Study the drawing (mm; zero at the part's minimum x, y, z) and answer. Give positions to 0.01 mm unless a question says otherwise; leave off trailing zeros. Order: outer loops, then holes, each group sorted by start corner. A loop starts at its lowest first (then second) coordinate and runs counter-clockwise, first axis right, second up. Notation, with made-up numbers: (0, 47) -> (19, 47) arc R25 cw to (19, 80) -> close; hole circle Ø2 at (-6.5, -3). An arc over 180 degrees is marked (long way). Answer as CSV lines item,"result". Start each with the question number.
1. A cutting plane is placed at A-A (y = 3.75). Give the vertices of the cut face in (x, z) (1 decimal).
2. Find the intervals of material crossed by L1, parallel to X at y = 5, z = 1.25; L2, parallel to Y at x = 2, z = 7.5 (1 decimal); L3, parallel to Y at x = 1, z = 2 (1 decimal), in increasing order.
3. A cutting plane is placed at D-D (y = 5.25). Give the vertices of the cut face in (x, z).
4. A cutting plane is placed at B-B (x = 9). Give the vertices of the cut face in (y, z) (1 decimal).
5. A cutting plane is placed at C-C (z = 8.25). Give the vertices of the cut face in (x, y) (1 decimal).
6. For a pull along X with two mould halves and no side action, classify the marked faces 1, 2 and 3 as released by +X, released by -X, zero draft, split by the parting line, or undercut.
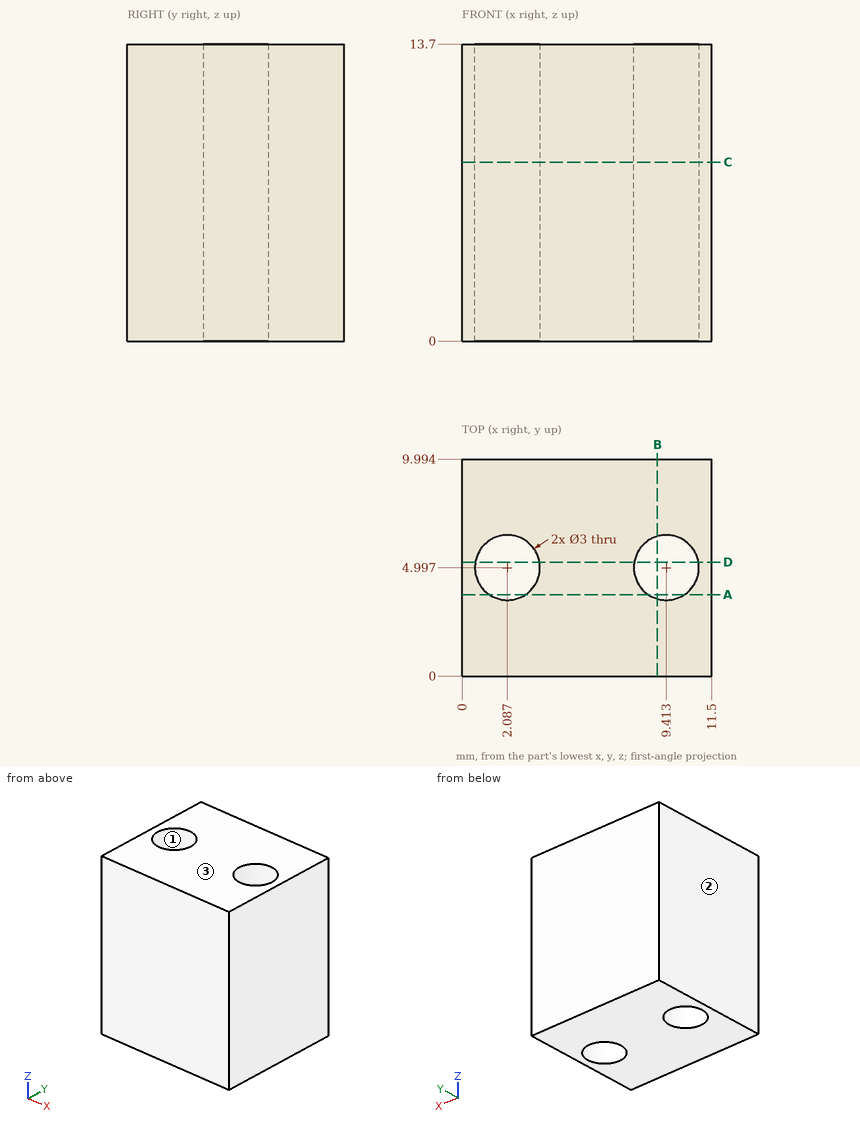
Answer sheet:
1,outline,"(0, 0) -> (1.3, 0) -> (1.3, 13.7) -> (0, 13.7) -> close; (2.9, 0) -> (8.6, 0) -> (8.6, 13.7) -> (2.9, 13.7) -> close; (10.2, 0) -> (11.5, 0) -> (11.5, 13.7) -> (10.2, 13.7) -> close"
2,L1,"x = 0 to 0.59, 3.59 to 7.91, 10.91 to 11.5"
2,L2,"y = 0 to 3.5, 6.5 to 10"
2,L3,"y = 0 to 4, 6 to 10"
3,outline,"(0, 0) -> (0.61, 0) -> (0.61, 13.7) -> (0, 13.7) -> close; (3.57, 0) -> (7.93, 0) -> (7.93, 13.7) -> (3.57, 13.7) -> close; (10.89, 0) -> (11.5, 0) -> (11.5, 13.7) -> (10.89, 13.7) -> close"
4,outline,"(0, 0) -> (3.6, 0) -> (3.6, 13.7) -> (0, 13.7) -> close; (6.4, 0) -> (10, 0) -> (10, 13.7) -> (6.4, 13.7) -> close"
5,outline,"(0, 0) -> (11.5, 0) -> (11.5, 10) -> (0, 10) -> close; hole circle Ø3 at (2.1, 5); hole circle Ø3 at (9.4, 5)"
6,face 1,"undercut"
6,face 2,"released by -X"
6,face 3,"zero draft"
